For this review, take the finished solid that the model builds, in its own axes (mm). A direction names the side the tool comes from. Give positions to 0.01 mm unless a question says otherwise; leave off trailing zeros. Order: outer loops, then holes, each group sorted by start corner. A loop starts at its lowest first (then second) coordinate and runs counter-clockwise, first axis right, second up. Notation, with made-up numbers: M 74.5,26.25 L 80.5,26.25 A36 cw 80.5,62.25 Z; hole C 44,41 d2. An arc over 180 degrees is marked long. Use CSV: the item, a comma, the result in double quotes. Start each with the question number.
(1) Wall thickness on L1, parallel to Z at x = 16, y = 1.45; L2, parallel to X at y = 0.5, z = 22: over which ranges is each line inside the solid? List them lowest first. Write a range as from..to.
(2) Tool access review of faces 1 (the face through (40, 1, 37.74)), 2 (the face through (12, 1, -45.5)), 3 (the face through (-39, 1, 21)), 4 (the face through (-39, 1, -42)), 5 (the face through (-30, 1, 47)): name each direction out of +Z, -Z, +X, -X, +Y, -Y from which nothing blocks a thin tool from reaching the whole face with its end or side.
(3) Consider section A-A (z = 4). Write out the cut boundary in (x, y), and give its area (3 significant figures).
(4) Consider section B-B (x = 35). Write out the cut boundary in (y, z).
(5) Clearance check with flat-ended pins moving along their axes: P1, Ø0.9, axis at y = 1.5, z = -1.5, coming from the +X side; P2, Ø6, axis at x = 1.5, z = -15.5, coming from the -Y side; P3, Ø1.5, axis at y = 2, z = -47, coming from the -X side; P4, Ø0.9, axis at y = 1.5, z = -20, coming from the -X side. State where each tip first meets the part, or that it passes through.
(6) Draft analysis for pull direction Z (two halves, no side actions). For faces 6 (the face through (-41, 1, 26.958)), 7 (the face through (-1, 3, -1)), 8 (the face through (40, 1, -37.722)), 9 (the face through (-41, 1, 16.18)), state which applies: pulls with the +Z half, pulls with the -Z half, needs draft (parallel to the pull), parting line crosses it, or undercut.
```python
from build123d import *

# Parameters (mm, degrees)
ESBO_O1_W                = 84
ESBO_O1_H                = 97
RESSALTO_EXTRUS_O1_DEPTH = 3
ESBO_O2_W                = 3
ESBO_O2_H                = 10.777777778
CORTE_EXTRUS_O4_DEPTH    = 3
CORTE_EXTRUS_O9_REACH    = 66.228
ESBO_O5_W                = 12
ESBO_O5_H                = 3


with BuildPart() as part:
    # Esboço1 → Ressalto-extrusão1 (new body)
    with BuildSketch(Plane(origin=(0, 0, 0), x_dir=(1, 0, 0), z_dir=(0, 1, 0))):
        Rectangle(ESBO_O1_W, ESBO_O1_H)
    extrude(amount=RESSALTO_EXTRUS_O1_DEPTH)

    # Esboço2 → Corte-extrusão4 (cut)
    with BuildSketch(Plane.XZ):
        with Locations((-40.5, -43.111111111)):
            Rectangle(ESBO_O2_W, ESBO_O2_H)
        with Locations((40.5, -43.111111111)):
            Rectangle(ESBO_O2_W, ESBO_O2_H)
        with Locations((40.5, -21.551111111)):
            Rectangle(ESBO_O2_W, ESBO_O2_H)
        with Locations((40.5, 0.008888889)):
            Rectangle(ESBO_O2_W, ESBO_O2_H)
        with Locations((40.5, 21.568888889)):
            Rectangle(ESBO_O2_W, ESBO_O2_H)
        with Locations((40.5, 43.128888889)):
            Rectangle(ESBO_O2_W, ESBO_O2_H)
        with Locations((-40.5, -21.551111111)):
            Rectangle(ESBO_O2_W, ESBO_O2_H)
        with Locations((-40.5, 0.008888889)):
            Rectangle(ESBO_O2_W, ESBO_O2_H)
        with Locations((-40.5, 21.568888889)):
            Rectangle(ESBO_O2_W, ESBO_O2_H)
        with Locations((-40.5, 43.128888889)):
            Rectangle(ESBO_O2_W, ESBO_O2_H)
    extrude(amount=-CORTE_EXTRUS_O4_DEPTH, mode=Mode.SUBTRACT)

    # Esboço5 → Corte-extrusão9 (cut, up to next)
    with BuildSketch(Plane(origin=(0, 0, 0), x_dir=(1, 0, 0), z_dir=(0, 1, 0)), mode=Mode.PRIVATE) as corte_extrus_o9_sk1:
        with Locations((-36, 47)):
            Rectangle(ESBO_O5_W, ESBO_O5_H)
    corte_extrus_o9_tool1 = extrude(corte_extrus_o9_sk1.sketch, amount=CORTE_EXTRUS_O9_REACH, mode=Mode.PRIVATE) & part.part
    # Esboço5 → Corte-extrusão9 (cut, up to next)
    with BuildSketch(Plane(origin=(0, 0, 0), x_dir=(1, 0, 0), z_dir=(0, 1, 0)), mode=Mode.PRIVATE) as corte_extrus_o9_sk2:
        with Locations((-36, -47)):
            Rectangle(ESBO_O5_W, ESBO_O5_H)
    corte_extrus_o9_tool2 = extrude(corte_extrus_o9_sk2.sketch, amount=CORTE_EXTRUS_O9_REACH, mode=Mode.PRIVATE) & part.part
    # Esboço5 → Corte-extrusão9 (cut, up to next)
    with BuildSketch(Plane(origin=(0, 0, 0), x_dir=(1, 0, 0), z_dir=(0, 1, 0)), mode=Mode.PRIVATE) as corte_extrus_o9_sk3:
        with Locations((36, -47)):
            Rectangle(ESBO_O5_W, ESBO_O5_H)
    corte_extrus_o9_tool3 = extrude(corte_extrus_o9_sk3.sketch, amount=CORTE_EXTRUS_O9_REACH, mode=Mode.PRIVATE) & part.part
    # Esboço5 → Corte-extrusão9 (cut, up to next)
    with BuildSketch(Plane(origin=(0, 0, 0), x_dir=(1, 0, 0), z_dir=(0, 1, 0)), mode=Mode.PRIVATE) as corte_extrus_o9_sk4:
        with Locations((36, 47)):
            Rectangle(ESBO_O5_W, ESBO_O5_H)
    corte_extrus_o9_tool4 = extrude(corte_extrus_o9_sk4.sketch, amount=CORTE_EXTRUS_O9_REACH, mode=Mode.PRIVATE) & part.part
    # Esboço5 → Corte-extrusão9 (cut, up to next)
    with BuildSketch(Plane(origin=(0, 0, 0), x_dir=(1, 0, 0), z_dir=(0, 1, 0)), mode=Mode.PRIVATE) as corte_extrus_o9_sk5:
        with Locations((-12, -47)):
            Rectangle(ESBO_O5_W, ESBO_O5_H)
    corte_extrus_o9_tool5 = extrude(corte_extrus_o9_sk5.sketch, amount=CORTE_EXTRUS_O9_REACH, mode=Mode.PRIVATE) & part.part
    # Esboço5 → Corte-extrusão9 (cut, up to next)
    with BuildSketch(Plane(origin=(0, 0, 0), x_dir=(1, 0, 0), z_dir=(0, 1, 0)), mode=Mode.PRIVATE) as corte_extrus_o9_sk6:
        with Locations((12, -47)):
            Rectangle(ESBO_O5_W, ESBO_O5_H)
    corte_extrus_o9_tool6 = extrude(corte_extrus_o9_sk6.sketch, amount=CORTE_EXTRUS_O9_REACH, mode=Mode.PRIVATE) & part.part
    # Esboço5 → Corte-extrusão9 (cut, up to next)
    with BuildSketch(Plane(origin=(0, 0, 0), x_dir=(1, 0, 0), z_dir=(0, 1, 0)), mode=Mode.PRIVATE) as corte_extrus_o9_sk7:
        with Locations((-12, 47)):
            Rectangle(ESBO_O5_W, ESBO_O5_H)
    corte_extrus_o9_tool7 = extrude(corte_extrus_o9_sk7.sketch, amount=CORTE_EXTRUS_O9_REACH, mode=Mode.PRIVATE) & part.part
    # Esboço5 → Corte-extrusão9 (cut, up to next)
    with BuildSketch(Plane(origin=(0, 0, 0), x_dir=(1, 0, 0), z_dir=(0, 1, 0)), mode=Mode.PRIVATE) as corte_extrus_o9_sk8:
        with Locations((12, 47)):
            Rectangle(ESBO_O5_W, ESBO_O5_H)
    corte_extrus_o9_tool8 = extrude(corte_extrus_o9_sk8.sketch, amount=CORTE_EXTRUS_O9_REACH, mode=Mode.PRIVATE) & part.part
    add(corte_extrus_o9_tool1.solids().sort_by_distance((-36, 0, -47))[0], mode=Mode.SUBTRACT)
    add(corte_extrus_o9_tool2.solids().sort_by_distance((-36, 0, 47))[0], mode=Mode.SUBTRACT)
    add(corte_extrus_o9_tool3.solids().sort_by_distance((36, 0, 47))[0], mode=Mode.SUBTRACT)
    add(corte_extrus_o9_tool4.solids().sort_by_distance((36, 0, -47))[0], mode=Mode.SUBTRACT)
    add(corte_extrus_o9_tool5.solids().sort_by_distance((-12, 0, 47))[0], mode=Mode.SUBTRACT)
    add(corte_extrus_o9_tool6.solids().sort_by_distance((12, 0, 47))[0], mode=Mode.SUBTRACT)
    add(corte_extrus_o9_tool7.solids().sort_by_distance((-12, 0, -47))[0], mode=Mode.SUBTRACT)
    add(corte_extrus_o9_tool8.solids().sort_by_distance((12, 0, -47))[0], mode=Mode.SUBTRACT)


solid = part.part
```
Check result:
1,L1,"z = -45.5..45.5"
1,L2,"x = -39..39"
2,face 1,"+Z, +X, +Y, -Y"
2,face 2,"-Z, +Y, -Y"
2,face 3,"-X, +Y, -Y"
2,face 4,"-Z, -X, +Y, -Y"
2,face 5,"+Z, -X, +Y, -Y"
3,outline,"M -39,0 L 39,0 L 39,3 L -39,3 Z"
3,area,"234 mm^2"
4,outline,"M 0,-45.5 L 3,-45.5 L 3,45.5 L 0,45.5 Z"
5,P1,"stops at x = 39"
5,P2,"stops at y = 0"
5,P3,"stops at x = -30"
5,P4,"stops at x = -39"
6,face 6,"undercut"
6,face 7,"needs draft"
6,face 8,"pulls with the -Z half"
6,face 9,"undercut"
